Can you work these out from the model? Positions are in its coordinate system, mm. Coordinates: 2 decimals unless noted, no trailing zeros. Order: outer loops, then holes, each group sorted by start corner. A loop starts at its lowest first (then second) coordinate and runs counter-clockwise, first axis right, second up. Notation, with made-up numbers: (86.25, 12.25) - (119.25, 12.25) arc R26 ccw to (119.25, 43.25) - close; hole circle Ø10 at (-35.75, -8.75). An arc over 180 degrees is marked (long way). Return JSON: item names as keys, results as strings. Group by question number.
1) Imagine slicing it at B-B (y = 102). Write out the boundary of the cut face in (x, z) (3 decimals), and give its area (3 significant figures).
2) If I drill on line 1 along X through (y, z) = (-90, 1.2); line 2 along Y through (x, z) = (-179, 2.1), over which ranges is the centre line in solid material (lowest first)?
3) Imagine slicing it at C-C (z = 2.6). Give the number of separate pieces and of enclosed holes in the cut face, and give its area (3 significant figures).
4) Imagine slicing it at A-A (x = -91.5). Write out the boundary of the cut face in (y, z) (3 decimals).
5) For pin 1 Ø1 at (x, y) = (-85.5, -109.5) entering from +Z, with a flat end and sliding along its axis, tell me the tip position at first contact or that it passes through.
```python
from build123d import *

# Parameters (mm, degrees)
SKETCH1_W           = 441.979400076
SKETCH1_H           = 305.81676
BOSS_EXTRUDE1_DEPTH = 3.175
CUT_EXTRUDE1_DEPTH  = 271.654843319
CUT_EXTRUDE2_DEPTH  = 271.654843319
LPATTERN1_COUNT     = 3
LPATTERN1_PITCH     = 181.613999992
LPATTERN2_COUNT     = 2
LPATTERN2_PITCH     = 181.613999992


with BuildPart() as part:
    # Sketch1 → Boss-Extrude1 (new body)
    with BuildSketch(Plane.XY):
        with Locations((0, -3.32067)):
            Rectangle(SKETCH1_W, SKETCH1_H)
    extrude(amount=BOSS_EXTRUDE1_DEPTH)

    # Sketch2 → Cut-Extrude1 (cut, through all)
    with BuildSketch(Plane.XY.offset(3.175)):
        with BuildLine():
            Line((-185.746625, -116.8), (-166.696625, -116.8))
            ThreePointArc((-166.696625, -116.8), (-164.45156097, -115.87006403), (-163.521625, -113.625))
            Line((-163.521625, -113.625), (-163.521625, -81.875))
            ThreePointArc((-163.521625, -81.875), (-164.45156097, -79.62993597), (-166.696625, -78.7))
            Line((-166.696625, -78.7), (-185.746625, -78.7))
            ThreePointArc((-185.746625, -78.7), (-187.99168903, -79.62993597), (-188.921625, -81.875))
            Line((-188.921625, -81.875), (-188.921625, -113.625))
            ThreePointArc((-188.921625, -113.625), (-187.99168903, -115.87006403), (-185.746625, -116.8))
        make_face()
        with BuildLine():
            Line((-185.746625, 78.7), (-166.696625, 78.7))
            ThreePointArc((-166.696625, 78.7), (-164.45156097, 79.62993597), (-163.521625, 81.875))
            Line((-163.521625, 81.875), (-163.521625, 113.625))
            ThreePointArc((-163.521625, 113.625), (-164.45156097, 115.87006403), (-166.696625, 116.8))
            Line((-166.696625, 116.8), (-185.746625, 116.8))
            ThreePointArc((-185.746625, 116.8), (-187.99168903, 115.87006403), (-188.921625, 113.625))
            Line((-188.921625, 113.625), (-188.921625, 81.875))
            ThreePointArc((-188.921625, 81.875), (-187.99168903, 79.62993597), (-185.746625, 78.7))
        make_face()
    cut_extrude1 = extrude(amount=-CUT_EXTRUDE1_DEPTH, mode=Mode.SUBTRACT)

    # Sketch3 → Cut-Extrude2 (cut, through all)
    with BuildSketch(Plane.XY.offset(3.175)):
        with BuildLine():
            Line((-108.906375, -81.875), (-108.906375, -113.625))
            ThreePointArc((-108.906375, -113.625), (-107.97643903, -115.87006403), (-105.731375, -116.8))
            Line((-105.731375, -116.8), (-86.681375, -116.8))
            ThreePointArc((-86.681375, -116.8), (-84.43631097, -115.87006403), (-83.506375, -113.625))
            Line((-83.506375, -113.625), (-83.506375, -81.875))
            ThreePointArc((-83.506375, -81.875), (-84.43631097, -79.62993597), (-86.681375, -78.7))
            Line((-86.681375, -78.7), (-105.731375, -78.7))
            ThreePointArc((-105.731375, -78.7), (-107.97643903, -79.62993597), (-108.906375, -81.875))
        make_face()
        with BuildLine():
            Line((-83.506375, 81.875), (-83.506375, 113.625))
            ThreePointArc((-83.506375, 113.625), (-84.43631097, 115.87006403), (-86.681375, 116.8))
            Line((-86.681375, 116.8), (-105.731375, 116.8))
            ThreePointArc((-105.731375, 116.8), (-107.97643903, 115.87006403), (-108.906375, 113.625))
            Line((-108.906375, 113.625), (-108.906375, 81.875))
            ThreePointArc((-108.906375, 81.875), (-107.97643903, 79.62993597), (-105.731375, 78.7))
            Line((-105.731375, 78.7), (-86.681375, 78.7))
            ThreePointArc((-86.681375, 78.7), (-84.43631097, 79.62993597), (-83.506375, 81.875))
        make_face()
    cut_extrude2 = extrude(amount=-CUT_EXTRUDE2_DEPTH, mode=Mode.SUBTRACT)

    # LPattern1: Cut-Extrude1 ×3
    with Locations(*[(i * LPATTERN1_PITCH, 0, 0) for i in range(1, LPATTERN1_COUNT)]):
        add(cut_extrude1, mode=Mode.SUBTRACT)

    # LPattern2: Cut-Extrude2 ×2
    with Locations(*[(i * LPATTERN2_PITCH, 0, 0) for i in range(1, LPATTERN2_COUNT)]):
        add(cut_extrude2, mode=Mode.SUBTRACT)


solid = part.part
```
Calculated:
{
 "1": {"outline": "(-220.99, 0) - (-188.922, 0) - (-188.922, 3.175) - (-220.99, 3.175) - close; (-163.522, 0) - (-108.906, 0) - (-108.906, 3.175) - (-163.522, 3.175) - close; (-83.506, 0) - (-7.308, 0) - (-7.308, 3.175) - (-83.506, 3.175) - close; (18.092, 0) - (72.708, 0) - (72.708, 3.175) - (18.092, 3.175) - close; (98.108, 0) - (174.306, 0) - (174.306, 3.175) - (98.108, 3.175) - close; (199.706, 0) - (220.99, 0) - (220.99, 3.175) - (199.706, 3.175) - close", "area": "1,000 mm2"},
 "2": {"line 1": "-220.99 to -188.92, -163.52 to -108.91, -83.51 to -7.31, 18.09 to 72.71, 98.11 to 174.31, 199.71 to 220.99", "line 2": "-156.23 to -116.8, -78.7 to 78.7, 116.8 to 149.59"},
 "3": {"separate pieces": "1", "enclosed holes": "10", "area": "126,000 mm2"},
 "4": {"outline": "(-156.229, 0) - (-116.8, 0) - (-116.8, 3.175) - (-156.229, 3.175) - close; (-78.7, 0) - (78.7, 0) - (78.7, 3.175) - (-78.7, 3.175) - close; (116.8, 0) - (149.588, 0) - (149.588, 3.175) - (116.8, 3.175) - close"},
 "5": {"pin 1": "through"}
}
